Design review of the part built by this model. Coordinates are the model's own, in mm. Face numbers are marked on the shaded views. A direction names the side the tool comes from. Round coordinates to 2 decimals unless told otherwise and drop trailing zeros. Loops run counter-clockwise (first coordinate to the right, second up) from the corner with the lowest first, then second, coordinate; pieces in that order, holes last. Notation, with made-up numbers: M 81,87 L 133,87 A33 cw 133,118 Z; hole C 2,68.25 d4. An arc over 180 degrees is marked long. Use a Markdown table: item, result.
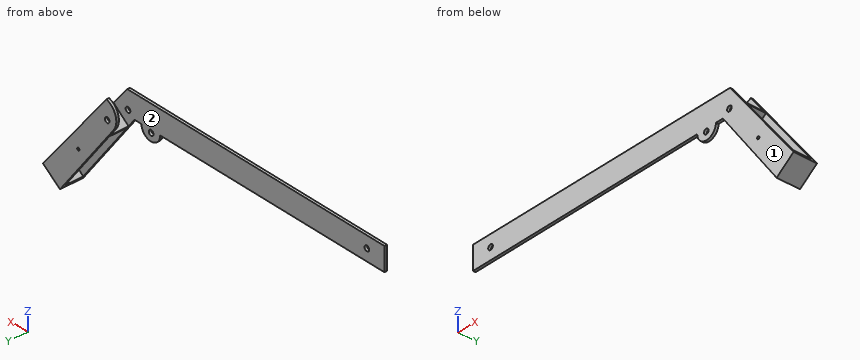
from build123d import *

# Parameters (mm, degrees)
F1_DEPTH  = 9
F3_DEPTH  = 8
F4_W      = 7
F4_H      = 42.4595763843
F4_H_2    = 6.157477504
F5_DEPTH  = 111.888617615
F7_DEPTH  = 9
F8_R      = 1
F8_R_2    = 0.5
F9_DEPTH  = 9.001
F10_R     = 1
F11_DEPTH = 9.001


# Not quite as in the source:
# - a feature names something its author has since deleted; it is built from what else it names


with BuildPart() as f1:
    # F0 (on Front) → F1 (new body)
    with BuildSketch(Plane.XZ):
        Polygon((-64.9861803949, 9), (-64.9861803949, 0), (31.0138196051, 0), (39.0138196051, 0), (42.0138196051, 0), (65.0138196051, -31.496031496), (72.2821345657, -26.1883391884), (45.1079792442, 9), align=None)
        with BuildLine():
            Line((39.0138196051, 0), (31.0138196051, 0))
            ThreePointArc((31.0138196051, 0), (35.0138196051, -4), (39.0138196051, 0))
        make_face()
    extrude(amount=F1_DEPTH)

    # F2 (on face) → F3 (cut)
    with BuildSketch(Plane(origin=(0, 0, 0), x_dir=(-1, 0, 0), z_dir=(0, 1, 0))):
        with BuildLine():
            ThreePointArc((-45.1079792442, 9), (-41.2127769921, 5.307273962), (-42.0138196051, 0))
            Line((-42.0138196051, 0), (-39.0138196051, 0))
            ThreePointArc((-39.0138196051, 0), (-35.0138196051, -4), (-31.0138196051, 0))
            Line((-31.0138196051, 0), (64.9861803949, 0))
            Line((64.9861803949, 0), (64.9861803949, 9))
            Line((64.9861803949, 9), (-45.1079792442, 9))
        make_face()
    extrude(amount=-F3_DEPTH, mode=Mode.SUBTRACT)

    # F4 (on face) → F5 (cut, through all)
    with BuildSketch(Plane(origin=(32.6104059702, 0, 25.1833492962), x_dir=(0, 1, 0), z_dir=(0.7914681616, 0, 0.6112103968))):
        with Locations((-4.5, -41.6770406282)):
            Rectangle(F4_W, F4_H)
        with Locations((-4.5, -17.368513684)):
            Rectangle(F4_W, F4_H_2)
    extrude(amount=-F5_DEPTH, mode=Mode.SUBTRACT)

    # F6 (on face) → F7 (join)
    with BuildSketch(Plane.XZ.offset(9)):
        Polygon((45.0138196051, -4.1081780212), (51.5466572041, 0.662431406), (50.9354468073, 1.4538995677), (44.551974041, -3.4757300893), align=None)
    extrude(amount=-F7_DEPTH)

    # F8 (on face) → F9 (cut, through all)
    with BuildSketch(Plane.XZ.offset(9)):
        with Locations((44.8008679783, 2.0352441098)):
            Circle(F8_R)
        with Locations((57.1549696039, -13.9623209745)):
            Circle(F8_R_2)
        with Locations((-57.4861803949, 4.5)):
            Circle(F8_R)
    extrude(amount=-F9_DEPTH, mode=Mode.SUBTRACT)

    # F10 (on face) → F11 (cut, through all)
    with BuildSketch(Plane.XZ.offset(9)):
        with Locations((-60.9861803949, -1.4662119793)):
            Circle(F10_R)
        with Locations((34.8888196051, -0.9921567416)):
            Circle(F10_R)
    extrude(amount=-F11_DEPTH, mode=Mode.SUBTRACT)


solid = f1.part
1. Take a section at A-A on y = -4.75. Give the boundary of the cut face in (x, z), and give its area (3 significant figures).
Check values:
| item | result |
|---|---|
| outline | M 44.55,-3.48 L 45.01,-4.11 L 51.55,0.66 L 50.94,1.45 Z; M 63.98,-30.08 L 65.01,-31.5 L 72.28,-26.19 L 71.06,-24.61 Z |
| area | 24.1 mm² |
2. Machinability: for the marked faces 1 and 2, which of the approach directions +Z, -Z, +X, -X, +Y, -Y give a long, thin tool a straight path to every point of the face, cutting with its end or side? Answer none if there is none.
Check values:
| item | result |
|---|---|
| face 1 | +Z, -Z, +X, -X, -Y |
| face 2 | +Z, -X |
3. Take a section at B-B on x = -23. Give the boundary of the cut face in (y, z), and give its area (3 significant figures).
Check values:
| item | result |
|---|---|
| outline | M -9,0 L -8,0 L -8,9 L -9,9 Z |
| area | 9.00 mm² |
4. Wall thickness on line 1 along Y through (x, z) = (40, 4); line 2 along X through (y, z) = (-0.5, 1.5); line 3 along X through (y, z) = (-0.75, -25): over which ranges is each line inside the solid? List them lowest first. Write a range as from..to.
Check values:
| item | result |
|---|---|
| line 1 | y = -9..-8 |
| line 2 | x = 41.22..43.96, 45.65..50.9 |
| line 3 | x = 60.27..71.36 |
5. Insertion check: pin 1 (6.5 mm diameter, centred on x = -7.5, z = 1.5, fed in from +Y); pin 2 (1.1 mm diameter, centred on x = 41, y = -8.5, fed in from -Z). Each pin has a flat end and moves straight along its axis. Give the tip position at first contact, or say it passes through.
Check values:
| item | result |
|---|---|
| pin 1 | stops at y = -8 |
| pin 2 | stops at z = 0 |
